CAD build for the part. Positions are in the model's coordinates, mm. A direction names the side the tool comes from. Round coordinates to 2 decimals unless told otherwise and drop trailing zeros. Loops run counter-clockwise (first coordinate to the right, second up) from the corner with the lowest first, then second, coordinate; pieces in that order, holes last. Notation, with made-up numbers: M 48.25,88.25 L 106.25,88.25 A25 ccw 106.25,103.25 Z; hole C -17,-23 d8. An arc over 180 degrees is marked long. Use a Markdown table: item, result. Add a question column.
(1) Which spindle directions (+Z, -Z, +X, -X, +Y, -Y) get a long thin tool onto all of the face, cutting with end or side? Do faces 1 (the face through (1.61, 26.74, 65.6)), 2 (the face through (27, 3.175, 50)). Say none if no direction does.
(2) Two-plate mould, pull along Z, no slides. Class faces 3 (the face through (1.61, 36.265, 65.182)), 4 (the face through (14, 3, 0)), 5 (the face through (14, 3, 101.6)): released by +Z, released by -Z, zero draft, split by the parting line, or undercut.
(3) Band-saw the part on A-A, the plane x = 25.4. Write the cut outline in (y, z) (3 decimals).
(4) Flat gauge pins, fed straight in: P1, Ø4, axis at x = 25, z = 75.5, coming from the +Y side (3 decimals); P2, Ø3, axis at x = 25.4, z = 63.5, coming from the +Y side; P3, Ø14.5, axis at y = 30, z = 63, coming from the +X side (3 decimals). Where does each tip first touch, or does it go through?
(5) Wall check: L1, parallel to Z at x = 25.4, y = 2.1; L2, parallel to X at y = 1, z = 63; L3, parallel to Z at x = 26.5, y = 3. Give the ranges that are in metal, low to high.
(6) Band-saw the part on D-D, the plane z = 59. Write the cut outline in (x, y) (3 decimals).
(7) Band-saw the part on C-C, the plane z = 12.7. Write the cut outline in (x, y) (3 decimals), and give its area (3 significant figures).
from build123d import *

# Parameters (mm, degrees)
BOSS_EXTRUDE1_DEPTH = 101.6
SKETCH3_R           = 2.4892
CUT_EXTRUDE1_DEPTH  = 124.171996107
SKETCH4_R           = 2.4892
CUT_EXTRUDE2_DEPTH  = 124.171996107


with BuildPart() as part:
    # Sketch2 → Boss-Extrude1 (new body)
    with BuildSketch(Plane.XY):
        Polygon((0, 0), (0, 50.8), (3.175, 50.8), (3.175, 3.175), (50.8, 3.175), (50.8, 0), align=None)
    extrude(amount=BOSS_EXTRUDE1_DEPTH)

    # Sketch3 → Cut-Extrude1 (cut, through all)
    with BuildSketch(Plane(origin=(0, 3.175, 0), x_dir=(1, 0, 0), z_dir=(0, 1, 0))):
        with Locations(Location((25.4, -12.7, 0), (0, 0, 180))):
            Circle(SKETCH3_R)
        with Locations(Location((38.1, -12.7, 0), (0, 0, 180))):
            Circle(SKETCH3_R)
        with Locations(Location((38.1, -38.1, 0), (0, 0, 180))):
            Circle(SKETCH3_R)
        with Locations(Location((38.1, -63.5, 0), (0, 0, 180))):
            Circle(SKETCH3_R)
        with Locations(Location((38.1, -88.9, 0), (0, 0, 180))):
            Circle(SKETCH3_R)
        with Locations(Location((25.4, -38.1, 0), (0, 0, 180))):
            Circle(SKETCH3_R)
        with Locations(Location((25.4, -63.5, 0), (0, 0, 180))):
            Circle(SKETCH3_R)
        with Locations(Location((25.4, -88.9, 0), (0, 0, 180))):
            Circle(SKETCH3_R)
    extrude(amount=-CUT_EXTRUDE1_DEPTH, mode=Mode.SUBTRACT)

    # Sketch4 → Cut-Extrude2 (cut, through all)
    with BuildSketch(Plane(origin=(3.175, 0, 0), x_dir=(0, 0, -1), z_dir=(1, 0, 0))):
        with Locations(Location((-12.7, 25.4, 0), (0, 0, 90))):
            Circle(SKETCH4_R)
        with Locations(Location((-38.1, 25.4, 0), (0, 0, 90))):
            Circle(SKETCH4_R)
        with Locations(Location((-63.5, 25.4, 0), (0, 0, 90))):
            Circle(SKETCH4_R)
        with Locations(Location((-88.9, 25.4, 0), (0, 0, 90))):
            Circle(SKETCH4_R)
        with Locations(Location((-38.1, 38.1, 0), (0, 0, 90))):
            Circle(SKETCH4_R)
        with Locations(Location((-63.5, 38.1, 0), (0, 0, 90))):
            Circle(SKETCH4_R)
        with Locations(Location((-88.9, 38.1, 0), (0, 0, 90))):
            Circle(SKETCH4_R)
        with Locations(Location((-12.7, 38.1, 0), (0, 0, 90))):
            Circle(SKETCH4_R)
    extrude(amount=-CUT_EXTRUDE2_DEPTH, mode=Mode.SUBTRACT)


solid = part.part
Return value:
| question | item | result |
|---|---|---|
| 1 | face 1 | +X, -X |
| 1 | face 2 | +Z, -Z, +X, +Y |
| 2 | face 3 | undercut |
| 2 | face 4 | released by -Z |
| 2 | face 5 | released by +Z |
| 3 | outline | M 0,0 L 3.175,0 L 3.175,10.211 L 0,10.211 Z; M 0,15.189 L 3.175,15.189 L 3.175,35.611 L 0,35.611 Z; M 0,40.589 L 3.175,40.589 L 3.175,61.011 L 0,61.011 Z; M 0,65.989 L 3.175,65.989 L 3.175,86.411 L 0,86.411 Z; M 0,91.389 L 3.175,91.389 L 3.175,101.6 L 0,101.6 Z |
| 4 | P1 | y = 3.175 |
| 4 | P2 | through |
| 4 | P3 | x = 3.175 |
| 5 | L1 | 0 to 10.21, 15.19 to 35.61, 40.59 to 61.01, 65.99 to 86.41, 91.39 to 101.6 |
| 5 | L2 | 0 to 22.96, 27.84 to 35.66, 40.54 to 50.8 |
| 5 | L3 | 0 to 10.47, 14.93 to 35.87, 40.33 to 61.27, 65.73 to 86.67, 91.13 to 101.6 |
| 6 | outline | M 0,0 L 50.8,0 L 50.8,3.175 L 3.175,3.175 L 3.175,50.8 L 0,50.8 Z |
| 7 | outline | M 0,0 L 22.911,0 L 22.911,3.175 L 3.175,3.175 L 3.175,22.911 L 0,22.911 Z; M 0,27.889 L 3.175,27.889 L 3.175,35.611 L 0,35.611 Z; M 0,40.589 L 3.175,40.589 L 3.175,50.8 L 0,50.8 Z; M 27.889,0 L 35.611,0 L 35.611,3.175 L 27.889,3.175 Z; M 40.589,0 L 50.8,0 L 50.8,3.175 L 40.589,3.175 Z |
| 7 | area | 249 mm^2 |
